The model under review builds one solid part; all positions refer to its coordinate system, in mm. Round coordinates to 2 decimals unless told otherwise and drop trailing zeros. Order: outer loops, then holes, each group sorted by start corner. A loop starts at its lowest first (then second) coordinate and runs counter-clockwise, first axis right, second up. Notation, with made-up numbers: (-3.75, 1.5) - (35.25, 1.5) arc R21 cw to (35.25, 12.5) - close; hole circle Ø7 at (-29.5, 42.25). An arc over 180 degrees is marked (long way). One line per question, with ' | ' between items. Start each with the question number.
Item 1: For L1, parallel to X at y = -47.2, z = 0.1; L2, parallel to Y at x = 4.65, z = 0.1; L3, parallel to X at y = -12.5, z = 0.15 (3 decimals), list the stretches that pass through material, from the lowest coordinate up. Write a range as [from, to].
Item 2: Insertion check: pin 1 Ø4.5 at (x, y) = (4.65, -3.7) entering from +Z; pin 2 Ø2 at (x, y) = (4.65, -47.2) entering from -Z; pin 3 Ø4 at (x, y) = (120.15, -47.2) entering from +Z. Each pin has a flat end and moves straight along its axis. Give the tip position at first contact, or say it passes through.
Item 3: Add section A-A on z = 0.9. State the section outline as (x, y) points (3 decimals).
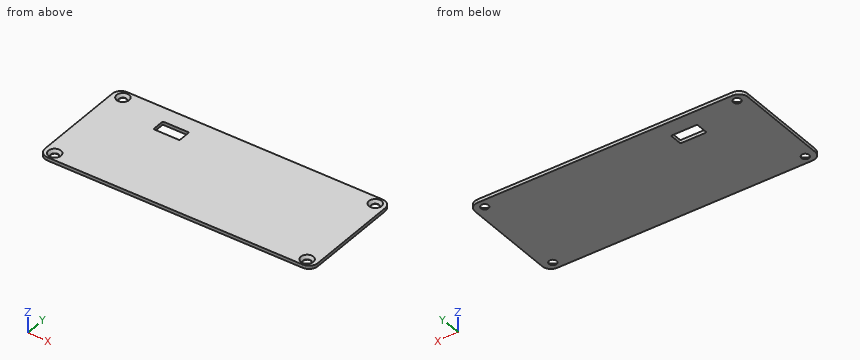
from build123d import *

# Parameters (mm, degrees)
SKETCH1_W                                      = 124.8
SKETCH1_H                                      = 50.9
SKETCH1_W_2                                    = 12
SKETCH1_H_2                                    = 6
BOSS_EXTRUDE1_DEPTH                            = 1.5
CSK_FOR_M3_5_FLAT_HEAD_MACHINE_SCREW1_AT_COUNT = 2
CSK_FOR_M3_5_FLAT_HEAD_MACHINE_SCREW1_AT_PITCH = 115.5
CSK_FOR_M3_5_FLAT_HEAD_MACHINE_SCREW_2_COUNT   = 2
CSK_FOR_M3_5_FLAT_HEAD_MACHINE_SCREW_2_PITCH   = 123.420014584
CSK_FOR_M3_5_FLAT_HEAD_MACHINE_SCREW_3_COUNT   = 2
CSK_FOR_M3_5_FLAT_HEAD_MACHINE_SCREW_3_PITCH   = 43.5
FILLET2_R                                      = 4
FILLET3_R                                      = 0.5


with BuildPart() as part:
    # Sketch1 → Boss-Extrude1 (new body)
    with BuildSketch(Plane.XY):
        with Locations((62.4, -25.45)):
            Rectangle(SKETCH1_W, SKETCH1_H)
        with Locations((31.565, -10.4)):
            Rectangle(SKETCH1_W_2, SKETCH1_H_2, mode=Mode.SUBTRACT)
    extrude(amount=BOSS_EXTRUDE1_DEPTH)

    # Sketch2 → CSK for M3.5 Flat Head Machine Screw1 (revolve, cut)
    with BuildSketch(Plane(origin=(4.65, -3.7, 1.5), x_dir=(0, -1, 0), z_dir=(1, 0, 0))):
        Polygon((0, 0), (0, 1.5), (1.75, 1.5), (1.75, 1.294164458), (2.875, 0), align=None)
    csk_for_m3_5_flat_head_machine_screw1 = revolve(axis=Axis((4.65, -3.7, 7.85), (0, 0, -1)), mode=Mode.SUBTRACT)

    # CSK for M3.5 Flat Head Machine Screw1 at: CSK for M3.5 Flat Head Machine Screw1 ×2
    with Locations(*[(i * CSK_FOR_M3_5_FLAT_HEAD_MACHINE_SCREW1_AT_PITCH, 0, 0) for i in range(1, CSK_FOR_M3_5_FLAT_HEAD_MACHINE_SCREW1_AT_COUNT)]):
        add(csk_for_m3_5_flat_head_machine_screw1, mode=Mode.SUBTRACT)

    # CSK for M3.5 Flat Head Machine Screw 2: CSK for M3.5 Flat Head Machine Screw1 ×2
    with Locations(*[Vector(0.935828766, -0.35245499, 0) * (i * CSK_FOR_M3_5_FLAT_HEAD_MACHINE_SCREW_2_PITCH) for i in range(1, CSK_FOR_M3_5_FLAT_HEAD_MACHINE_SCREW_2_COUNT)]):
        add(csk_for_m3_5_flat_head_machine_screw1, mode=Mode.SUBTRACT)

    # CSK for M3.5 Flat Head Machine Screw 3: CSK for M3.5 Flat Head Machine Screw1 ×2
    with Locations(*[(0, -i * CSK_FOR_M3_5_FLAT_HEAD_MACHINE_SCREW_3_PITCH, 0) for i in range(1, CSK_FOR_M3_5_FLAT_HEAD_MACHINE_SCREW_3_COUNT)]):
        add(csk_for_m3_5_flat_head_machine_screw1, mode=Mode.SUBTRACT)

    # Fillet2
    fillet2_edges = [part.edges().sort_by_distance(p)[0] for p in [
        (124.8, -50.9, 0.75),
        (0, -50.9, 0.75),
        (0, 0, 0.75),
        (124.8, 0, 0.75),
    ]]
    fillet(fillet2_edges, radius=FILLET2_R)

    # Fillet3
    fillet3_edges = [part.edges().sort_by_distance(p)[0] for p in [
        (25.565, -7.4, 0.75),
        (25.565, -13.4, 0.75),
        (37.565, -13.4, 0.75),
        (37.565, -7.4, 0.75),
    ]]
    fillet(fillet3_edges, radius=FILLET3_R)


solid = part.part
Determined:
1) L1: [0.01, 2.9], [6.4, 118.4], [121.9, 124.79] | L2: [-50.9, -48.95], [-45.45, -5.45], [-1.95, 0] | L3: [0, 25.565], [37.565, 124.8]
2) pin 1: z = 0.78 | pin 2: through | pin 3: z = 0.49
3) outline: (0, -46.9) arc R4 ccw to (4, -50.9) - (120.8, -50.9) arc R4 ccw to (124.8, -46.9) - (124.8, -4) arc R4 ccw to (120.8, 0) - (4, 0) arc R4 ccw to (0, -4) - close; hole circle Ø4.707 at (4.65, -47.2); hole circle Ø4.707 at (4.65, -3.7); hole (25.565, -12.9) arc R0.5 ccw to (26.065, -13.4) - (37.065, -13.4) arc R0.5 ccw to (37.565, -12.9) - (37.565, -7.9) arc R0.5 ccw to (37.065, -7.4) - (26.065, -7.4) arc R0.5 ccw to (25.565, -7.9) - close; hole circle Ø4.707 at (120.15, -47.2); hole circle Ø4.707 at (120.15, -3.7)
